The model under review builds one solid part; all positions refer to its coordinate system, in mm. A direction names the side the tool comes from. Coordinates: 2 decimals unless noted, no trailing zeros. Loops run counter-clockwise (first coordinate to the right, second up) from the corner with the lowest first, then second, coordinate; pieces in that order, holes last. Notation, with made-up numbers: (-6.75, 40) - (27.25, 40) arc R18 cw to (27.25, 72) - close; hole circle Ø3 at (29.25, 21). An arc over 180 degrees is marked (long way). Use a Markdown table: item, result. Add a question column.
1) Add section B-B, the plane z = 0. Give the boundary of the cut face in (x, y), and give its area (3 significant figures).
2) To check wall thickness, follow L1, parallel to X at y = 2.25, z = 0; L2, parallel to X at y = 2.2, z = 13.5; L3, parallel to X at y = 0.8, z = 7.5. State the ranges of each line that lie inside material, in increasing order. Write a range as [from, to].
3) Add section A-A, the plane x = -27.5. Give the boundary of the cut face in (y, z), and give its area (3 significant figures).
4) For faces 1 (the cylindrical face through (-25.914, 2.859, -0.208)), 2 (the cylindrical face through (23.24, 2.86, 16.12)), list the 3-axis set-ups (+Z, -Z, +X, -X, +Y, -Y) from which the entire face can be reached by the end or side of a thin tool; tool diameter is ignored.
5) Add section C-C, the plane z = 7.25. Give the boundary of the cut face in (x, y).
6) The part is to be moulded in two halves that separate along Z. For faces 3 (the cylindrical face through (21.93, 2.94, 4.6)), 4 (the cylindrical face through (-31.9, 2.94, -4.43)), 5 (the cylindrical face through (29.98, 2.86, 13.17)), say which applies: pulls with the +Z half, pulls with the -Z half, needs draft (parallel to the pull), parting line crosses it, or undercut.
7) Add section D-D, the plane y = 3.4. Give the boundary of the cut face in (x, z), and give its area (3 significant figures).
```python
from build123d import *

# Parameters (mm, degrees)
SKETCH_1_R      = 2.5
SKETCH_1_R_2    = 1.6
EXTRUDE_1_DEPTH = 5.8
FILLET_1_R      = 2


with BuildPart() as part:
    # ｽｹｯﾁ1 → ﾎﾞｽ - 押し出し1 (new body)
    with BuildSketch(Plane(origin=(0, 0, 0), x_dir=(1, 0, 0), z_dir=(0, 1, 0))):
        with BuildLine():
            ThreePointArc((29.679449472, -18), (31.736581603, -16.155442773), (32.5, -13.5))
            Line((32.5, -13.5), (32.5, -5))
            Line((32.5, -5), (32.5, 5))
            Line((32.5, 5), (-32.5, 5))
            Line((-32.5, 5), (-32.5, -5))
            Line((-32.5, -5), (-32.5, -13.5))
            ThreePointArc((-32.5, -13.5), (-31.736581603, -16.155442773), (-29.679449472, -18))
            Line((-29.679449472, -18), (-25.320550528, -18))
            ThreePointArc((-25.320550528, -18), (-23.263418397, -16.155442773), (-22.5, -13.5))
            Line((-22.5, -13.5), (-22.5, -4))
            Line((-22.5, -4), (22.5, -4))
            Line((22.5, -4), (22.5, -13.5))
            ThreePointArc((22.5, -13.5), (23.263418397, -16.155442773), (25.320550528, -18))
            Line((25.320550528, -18), (29.679449472, -18))
        make_face()
        with Locations(Location((-27.5, -13.5, 0), (0, 0, 270))):
            Circle(SKETCH_1_R, mode=Mode.SUBTRACT)
        with Locations(Location((27.5, -13.5, 0), (0, 0, 270))):
            Circle(SKETCH_1_R, mode=Mode.SUBTRACT)
        with Locations(Location((-27.5, 0, 0), (0, 0, 270))):
            Circle(SKETCH_1_R_2, mode=Mode.SUBTRACT)
        with Locations(Location((27.5, 0, 0), (0, 0, 270))):
            Circle(SKETCH_1_R_2, mode=Mode.SUBTRACT)
    extrude(amount=EXTRUDE_1_DEPTH)

    # ﾌｨﾚｯﾄ1
    fillet_1_edges = [part.edges().sort_by_distance(p)[0] for p in [
        (-32.5, 2.9, -5),
        (32.5, 2.9, -5),
        (22.5, 2.9, 4),
        (-22.5, 2.9, 4),
    ]]
    fillet(fillet_1_edges, radius=FILLET_1_R)


solid = part.part
```
From the geometry:
| question | item | result |
|---|---|---|
| 1 | outline | (-32.5, 0) - (-29.1, 0) - (-29.1, 5.8) - (-32.5, 5.8) - close; (-25.9, 0) - (25.9, 0) - (25.9, 5.8) - (-25.9, 5.8) - close; (29.1, 0) - (32.5, 0) - (32.5, 5.8) - (29.1, 5.8) - close |
| 1 | area | 340 mm^2 |
| 2 | L1 | x = [-32.5, -29.1], [-25.9, 25.9], [29.1, 32.5] |
| 2 | L2 | x = [-32.5, -30], [-25, -22.5], [22.5, 25], [30, 32.5] |
| 2 | L3 | x = [-32.5, -22.5], [22.5, 32.5] |
| 3 | outline | (0, -5) - (5.8, -5) - (5.8, -1.6) - (0, -1.6) - close; (0, 1.6) - (5.8, 1.6) - (5.8, 11) - (0, 11) - close; (0, 16) - (5.8, 16) - (5.8, 18) - (0, 18) - close |
| 3 | area | 85.8 mm^2 |
| 4 | face 1 | +Y, -Y |
| 4 | face 2 | +Z, +Y, -Y |
| 5 | outline | (-32.5, 0) - (-22.5, 0) - (-22.5, 5.8) - (-32.5, 5.8) - close; (22.5, 0) - (32.5, 0) - (32.5, 5.8) - (22.5, 5.8) - close |
| 6 | face 3 | pulls with the +Z half |
| 6 | face 4 | pulls with the -Z half |
| 6 | face 5 | undercut |
| 7 | outline | (-32.5, -3) arc R2 ccw to (-30.5, -5) - (30.5, -5) arc R2 ccw to (32.5, -3) - (32.5, 13.5) arc R5 ccw to (29.68, 18) - (25.32, 18) arc R5 ccw to (22.5, 13.5) - (22.5, 6) arc R2 cw to (20.5, 4) - (-20.5, 4) arc R2 cw to (-22.5, 6) - (-22.5, 13.5) arc R5 ccw to (-25.32, 18) - (-29.68, 18) arc R5 ccw to (-32.5, 13.5) - close; hole circle Ø5 at (-27.5, 13.5); hole circle Ø3.2 at (-27.5, 0); hole circle Ø5 at (27.5, 13.5); hole circle Ø3.2 at (27.5, 0) |
| 7 | area | 795 mm^2 |
